Check sheet for the modelled part. Datum: model origin and axes. Units: mm. A direction names the side the tool comes from. Coordinates: 2 decimals unless noted, no trailing zeros. Loops run counter-clockwise (first coordinate to the right, second up) from the corner with the lowest first, then second, coordinate; pieces in that order, holes last.
from build123d import *

# Parameters (mm, degrees)
SKETCH1_W            = 60
SKETCH1_H            = 60
BOSS_EXTRUDE1_DEPTH  = 60
CUT_EXTRUDE1_DEPTH   = 60
CUT_EXTRUDE2_DEPTH   = 60
CUT_EXTRUDE3_DEPTH   = 60
CUT_EXTRUDE4_DEPTH   = 60
CUT_EXTRUDE5_DEPTH   = 60
CUT_EXTRUDE6_DEPTH   = 60
CUT_EXTRUDE7_DEPTH   = 60
CUT_EXTRUDE8_DEPTH   = 60
BOSS_EXTRUDE3_DEPTH  = 60
BOSS_EXTRUDE7_DEPTH  = 0.15
BOSS_EXTRUDE8_DEPTH  = 0.15
CUT_EXTRUDE10_DEPTH  = 0.5
BOSS_EXTRUDE10_DEPTH = 0.0001


with BuildPart() as part:
    # Sketch1 → Boss-Extrude1 (new body)
    with BuildSketch(Plane.XY):
        with Locations((30, 30)):
            Rectangle(SKETCH1_W, SKETCH1_H)
    extrude(amount=BOSS_EXTRUDE1_DEPTH)

    # Sketch2 → Cut-Extrude1 (cut)
    with BuildSketch(Plane.XY.offset(60)):
        Polygon((30, 60), (0, 30), (0, 60), align=None)
    extrude(amount=-CUT_EXTRUDE1_DEPTH, mode=Mode.SUBTRACT)

    # Sketch3 → Cut-Extrude2 (cut)
    with BuildSketch(Plane(origin=(60, 0, 0), x_dir=(0, 0, -1), z_dir=(1, 0, 0))):
        Polygon((-60, 30), (-30, 60), (-60, 60), align=None)
    extrude(amount=-CUT_EXTRUDE2_DEPTH, mode=Mode.SUBTRACT)

    # Sketch4 → Cut-Extrude3 (cut)
    with BuildSketch(Plane(origin=(30, 60, 30), x_dir=(0.912870929, -0.365148372, -0.182574186), z_dir=(0.40824829, 0.816496581, 0.40824829))):
        Polygon((0, 0), (32.86335345, 26.83281573), (32.86335345, -40.249223595), align=None)
    extrude(amount=CUT_EXTRUDE3_DEPTH, mode=Mode.SUBTRACT)

    # Sketch5 → Cut-Extrude4 (cut)
    with BuildSketch(Plane(origin=(0, 24, 48), x_dir=(1, 0, 0), z_dir=(0, 0.447213595, 0.894427191))):
        Polygon((0, -26.83281573), (60, -26.83281573), (30, 40.249223595), align=None)
    extrude(amount=CUT_EXTRUDE4_DEPTH, mode=Mode.SUBTRACT)

    # Sketch6 → Cut-Extrude5 (cut)
    with BuildSketch(Plane(origin=(10, -4, 2), x_dir=(0.169515876, -0.06780635, -0.98319208), z_dir=(0.912870929, -0.365148372, 0.182574186))):
        Polygon((-58.991524815, 32.310988843), (-58.991524815, 0), (-28.478667152, 66.850321744), align=None)
    extrude(amount=-CUT_EXTRUDE5_DEPTH, mode=Mode.SUBTRACT)

    # Sketch7 → Cut-Extrude6 (cut)
    with BuildSketch(Plane(origin=(40, 16, -8), x_dir=(0.169515876, 0.06780635, 0.98319208), z_dir=(-0.912870929, -0.365148372, 0.182574186))):
        Polygon((38.649619706, 44.566881162), (69.162477369, -22.283440581), (69.162477369, 10.027548262), align=None)
    extrude(amount=-CUT_EXTRUDE6_DEPTH, mode=Mode.SUBTRACT)

    # Sketch8 → Cut-Extrude7 (cut)
    with BuildSketch(Plane(origin=(11.724137931, 4.689655172, 68), x_dir=(-0.985527457, 0.011663047, 0.169114179), z_dir=(-0.169515876, -0.06780635, -0.98319208))):
        Polygon((-36.808575777, 25.800784356), (-47.082262149, 27.800345143), (-48.984796662, 27.017107047), (-48.984796662, -4.128125497), align=None)
    extrude(amount=-CUT_EXTRUDE7_DEPTH, mode=Mode.SUBTRACT)

    # Sketch9 → Cut-Extrude8 (cut)
    with BuildSketch(Plane(origin=(-10, 4, 58), x_dir=(-0.985527457, -0.011663047, -0.169114179), z_dir=(0.169515876, -0.06780635, -0.98319208))):
        Polygon((-10.146850737, -4.128125497), (-10.146850737, 25.943133511), (-12.04938525, 27.800345143), (-22.323071622, 25.800784356), align=None)
    extrude(amount=-CUT_EXTRUDE8_DEPTH, mode=Mode.SUBTRACT)

    # Sketch11 → Boss-Extrude3 (add)
    with BuildSketch(Plane.XY.offset(60)):
        Polygon((0, 0), (30, 30), (60, 0), align=None)
    extrude(amount=-BOSS_EXTRUDE3_DEPTH)

    # Sketch12 → Boss-Extrude7 (add)
    with BuildSketch(Plane.ZY):
        Polygon((45, 30), (60, 0), (60, 30), align=None)
    extrude(amount=-BOSS_EXTRUDE7_DEPTH)

    # Sketch13 → Boss-Extrude8 (add)
    with BuildSketch(Plane(origin=(-15, 15, 0), x_dir=(0.707106781, 0.707106781, 0), z_dir=(-0.707106781, 0.707106781, 0))):
        Polygon((63.639610307, -30), (21.213203436, -60), (21.213203436, -45), align=None)
    extrude(amount=-BOSS_EXTRUDE8_DEPTH)

    # Sketch14 → Cut-Extrude10 (cut)
    with BuildSketch(Plane(origin=(0, 0, 0), x_dir=(-1, 0, 0), z_dir=(0, 0, -1))):
        with BuildLine():
            Line((-30, 30), (0, 30))
            Line((0, 30), (-30, 60))
            Line((-30, 60), (-60, 60))
            ThreePointArc((-60, 60), (-51.213203436, 38.786796564), (-30, 30))
        make_face()
    extrude(amount=-CUT_EXTRUDE10_DEPTH, mode=Mode.SUBTRACT)

    # Sketch15 → Boss-Extrude10 (add)
    with BuildSketch(Plane(origin=(60, 0, 0), x_dir=(0, 0, -1), z_dir=(1, 0, 0))):
        with BuildLine():
            Line((-27.89036592, 30.074267861), (-44.962866069, 30.074267861))
            Line((-44.962866069, 30.074267861), (-40, 40))
            Line((-40, 40), (0, 60))
            ThreePointArc((0, 60), (-8.053599129, 39.546259784), (-27.89036592, 30.074267861))
        make_face()
    extrude(amount=BOSS_EXTRUDE10_DEPTH)


solid = part.part
(1) Section check D-D, the plane y = 11.5. Enter the section's corners in (x, z).
(2) Set-up check for faces 1 (the face through (41, 60, 12)), 2 (the face through (18, 18, 54)), 3 (the face through (37, 45, 0.5)), 4 (the face through (41, 19, 54)): record each of +Z, -Z, +X, -X, +Y, -Y from which the full face is reachable in a straight line by a thin tool's end or side.
(3) Scan lines: line 1 along Y through (x, z) = (10, 13.5); line 2 along Y through (x, z) = (46, 56); line 3 along Z through (x, y) = (22, 27.5). Record each from-to range of solid material in increasing order.
(4) Gauge pin test, flat ends, axial feed: P1, Ø1.5, axis at y = 49, z = 11, coming from the -X side; P2, Ø9, axis at x = 16.5, y = 44.5, coming from the -Z side. Record the tip position at first contact, or that the pin passes through.
(5) Section check B-B, the plane x = 16.5. Enter the section's corners in (y, z), plus the area to 3 significant figures.
(6) Section check A-A, the plane y = 22. Enter the section's corners in (x, z), plus the area to 3 significant figures.
Determined:
1. outline: (0, 0) - (60, 0) - (60, 54.25) - (48.5, 54.25) - (48.5, 60) - (11.5, 60) - (11.5, 54.25) - (0.15, 54.25) - (0.15, 60) - (0, 60) - close
2. face 1: +Z, -Z, +X, -X, +Y
2. face 2: +Z, +Y
2. face 3: -Z, -X, +Y
2. face 4: +Z, +X, +Y
3. line 1: y = 0 to 40
3. line 2: y = 0 to 14
3. line 3: z = 0 to 46.25
4. P1: stops at x = 18.25
4. P2: stops at z = 0.5
5. outline: (0, 0) - (30, 0) - (30, 0.5) - (46.5, 0.5) - (46.5, 43.5) - (46.29, 43.61) - (46.29, 36.86) - (16.5, 51.75) - (16.5, 60) - (0, 60) - close
5. area: 2,310 mm2
6. outline: (0, 0) - (60, 0) - (60, 49) - (38, 49) - (38, 60) - (22, 60) - (22, 49) - (0.15, 49) - (0.15, 60) - (0, 60) - close
6. area: 3,120 mm2
